Autodesk Inventor part; units mm, degrees
ref_plane "Arbeitsebene1" through (-6, 0, 0) normal (1, 0, 0) x (0, 1, 0)
ref_plane "XZ Plane" through (0, 0, 0) normal (0, 1, 0) x (-1, 0, 0)
ref_plane "XY Plane" through (0, 0, 0) normal (0, 0, 1) x (1, 0, 0)
sketch "Skizze1" plane through (0, 0, 0) normal (0, 0, 1) x (1, 0, 0)
  circle A0 centre (0, 0) radius 6
  dimension "d0" = 12
extrude "Extrusion1" add sketch "Skizze1" along normal blind 15
sketch "Skizze2" plane through (0, 0, 15) normal (0, 0, 1) x (1, 0, 0)
  circle A0 centre (0, 0) radius 6
  circle A1 centre (0, 0) radius 4
  dimension "d3" = 8
extrude "Extrusion2" add sketch "Skizze2" along normal blind 20 contours A1
sketch "Skizze3" plane through (0, 0, 0) normal (0, 0, -1) x (-1, 0, 0)
  circle A0 centre (0, 0) radius 6
hole "Bohrung1" at (0, 0, 0) direction (0, 0, 1) diameter 5 depth 25 tip angle 118
ref_plane "Arbeitsebene1" through (-6, 0, 0) normal (1, 0, 0) x (0, 1, 0)
sketch "Skizze4" plane through (-6, 0, 0) normal (1, 0, 0) x (0, 1, 0)
  line L0 (-8.4, 0) -> (8.4, 0)
  line L1 (0, -3) -> (0, 18)
  point P0 (0, 0)
  point P1 (0, 10)
  dimension "d13" = 10
hole "Bohrung2" at (-6, 0, 10) direction (1, 0, 0) diameter 2.459 end up to surface
chamfer "Fase1" distance 1 angle 45 1 edges at (-4, 0, 35)
properties part number "13_0204_061"
Build history of the part. All positions in model axes, mm. A direction names the side the tool comes from. Round coordinates to 2 decimals unless told otherwise and drop trailing zeros. Write each loop counter-clockwise with the first axis right and the second up, starting at its lowest first coordinate (ties: lowest second). Pieces come first, ordered by that corner, then holes. Notation, with made-up numbers: M -33,-35.5 L -26,-35.5 A20 ccw -26,-30.5 Z; hole C -1.75,-13.5 d2. An arc over 180 degrees is marked long. Answer in a Markdown table with one row per item.
1. Probe L1, parallel to Y at x = 0, z = 17.25; L2, parallel to Y at x = 0, z = 5. List the from-to ranges inside material, lowest first. Write a range as [from, to].
Geometry check:
| item | result |
|---|---|
| L1 | [-4, -2.5], [2.5, 4] |
| L2 | [-6, -2.5], [2.5, 6] |
2. Flat gauge pins, fed straight in: P1, Ø1, axis at x = 3.5, y = 2, coming from the +Z side; P2, Ø1, axis at x = 3.5, y = -4, coming from the +Z side; P3, Ø4, axis at y = -1.5, z = 14.5, coming from the -X side; P4, Ø2, axis at x = -1, y = 0.5, coming from the -Z side. Where does each tip first touch, or does it go through?
Geometry check:
| item | result |
|---|---|
| P1 | z = 34.47 |
| P2 | z = 15 |
| P3 | x = -6 |
| P4 | z = 25.23 |
3. Saw through at A-A (z = 19.5). List the corners of the cut face in (x, y), and give its area (3 significant figures).
Geometry check:
| item | result |
|---|---|
| outline | C 0,0 d8; hole C 0,0 d5 |
| area | 30.6 mm2 |
4. Saw through at B-B (x = -4.75). List the corners of the cut face in (y, z).
Geometry check:
| item | result |
|---|---|
| outline | M -3.67,0 L 3.67,0 L 3.67,15 L -3.67,15 Z; hole C 0,10 d2.46 |
5. Which spindle directions (+Z, -Z, +X, -X, +Y, -Y) get a long thin tool onto all of the face, cutting with end or side? Do faces 1 (the face through (-4.06, -1.22, 9.84)), 2 (the face through (-1.42, -3.92, 15)), 3 (the face through (5.723, -1.802, 7.395)). Say none if no direction does.
Geometry check:
| item | result |
|---|---|
| face 1 | -X |
| face 2 | +Z |
| face 3 | +Z, -Z |
6. Saw through at C-C (z = 28). List the corners of the cut face in (x, y).
Geometry check:
| item | result |
|---|---|
| outline | C 0,0 d8 |
7. Saw through at D-D (y = 5). List the corners of the cut face in (x, z), and give its area (3 significant figures).
Geometry check:
| item | result |
|---|---|
| outline | M -3.32,0 L 3.32,0 L 3.32,15 L -3.32,15 Z |
| area | 99.5 mm2 |
8. Mould opens along Y. For faces 4 (the face through (0, 0, 35)), 5 (the face through (-0.867, 3.905, 24.367)), 6 (the face through (2.44, -0.54, 12.68)), 7 (the face through (0.13, 0.414, 26.241)) say: +Y half, -Y half, draft (parallel to the pull), parting line (faces both ways), or undercut.
Geometry check:
| item | result |
|---|---|
| face 4 | draft |
| face 5 | parting line |
| face 6 | undercut |
| face 7 | undercut |
